Geometry check sheet. Reference: the model listing, model coordinates, mm. Give positions to 0.01 mm unless a question says otherwise; leave off trailing zeros. Write each loop counter-clockwise with the first axis right and the second up, starting at its lowest first coordinate (ties: lowest second). Pieces come first, ordered by that corner, then holes. Notation, with made-up numbers: (20.25, 37.25) - (67.25, 37.25) arc R19 ccw to (67.25, 54.25) - close; hole circle Ø1 at (13.5, 51). An arc over 180 degrees is marked (long way). Use a Markdown table: item, result.
```python
from build123d import *

# Parameters (mm, degrees)
F0_W     = 966.540682
F0_H     = 100
F1_DEPTH = 22
F3_DEPTH = 22
F5_DEPTH = 25


with BuildPart() as f1:
    # F0 (on Front) → F1 (new body)
    with BuildSketch(Plane.XZ):
        Rectangle(F0_W, F0_H)
    extrude(amount=F1_DEPTH)

    # F2 (on face) → F3 (cut)
    with BuildSketch(Plane.XZ.offset(22)):
        Polygon((-400.924605, -50), (-483.270341, 50), (-483.270341, -50), align=None)
    extrude(amount=-F3_DEPTH, mode=Mode.SUBTRACT)

    # F4 (on face) → F5 (cut)
    with BuildSketch(Plane.XZ.offset(22)):
        Polygon((483.270341, -50), (483.270341, 50), (400.924605, 50), align=None)
    extrude(amount=-F5_DEPTH, mode=Mode.SUBTRACT)


solid = f1.part
```
1) Section check A-A on y = -12.5. Record the boundary of the cut face in (x, z).
Working result:
| item | result |
|---|---|
| outline | (-483.27, 50) - (-400.92, -50) - (483.27, -50) - (400.92, 50) - close |
2) Depth check by flat-ended pin: P1, Ø10, axis at y = -9, z = 27.5, coming from the +X side; P2, Ø2, axis at y = -6.5, z = -31.5, coming from the -X side; P3, Ø8, axis at y = -12, z = 7, coming from the +X side. Enter the tip coordinate at first touch or a pass-through.
Working result:
| item | result |
|---|---|
| P1 | stops at x = 423.57 |
| P2 | stops at x = -416.98 |
| P3 | stops at x = 439.63 |
3) Section check B-B on z = -30. Record the boundary of the cut face in (x, y), then the cut area to 3 significant figures.
Working result:
| item | result |
|---|---|
| outline | (-417.39, -22) - (466.8, -22) - (466.8, 0) - (-417.39, 0) - close |
| area | 19,500 mm² |
4) Material ranges on L1, parallel to X at y = -6.5, z = -44; L2, parallel to X at y = -12.75, z = -6; L3, parallel to Z at x = -432, y = -19.75, recorded low to high. Write a range as from..to.
Working result:
| item | result |
|---|---|
| L1 | x = -405.87..478.33 |
| L2 | x = -437.16..447.04 |
| L3 | z = -12.26..50 |
